Geometry check sheet. Reference: the model listing, model coordinates, mm. A direction names the side the tool comes from. Coordinates: 2 decimals unless noted, no trailing zeros. Order: outer loops, then holes, each group sorted by start corner. A loop starts at its lowest first (then second) coordinate and runs counter-clockwise, first axis right, second up. Notation, with made-up numbers: (77, 18) -> (118, 18) arc R16 cw to (118, 41) -> close; hole circle Ø8 at (-26, -24.75). An arc over 180 degrees is marked (long way). Answer as CSV lines item,"result". Start each with the question number.
from build123d import *

# Parameters (mm, degrees)
CROQUIS1_R                   = 3
SALIENTE_EXTRUIR1_DEPTH      = 5
SALIENTE_EXTRUIR2_DEPTH      = 16
SALIENTE_EXTRUIR3_DEPTH      = 3
SALIENTE_EXTRUIR3_DEPTH_BACK = 3
SALIENTE_EXTRUIR4_DEPTH      = 3
SALIENTE_EXTRUIR4_DEPTH_BACK = 3
REDONDEO1_R                  = 3


with BuildPart() as part:
    # Croquis1 → Saliente-Extruir1 (new body)
    with BuildSketch(Plane.XY):
        with BuildLine():
            Line((-8, 0), (-8, 45))
            Line((-8, 45), (8, 45))
            Line((8, 45), (8, 0))
            ThreePointArc((8, 0), (0, -8), (-8, 0))
        make_face()
        Circle(CROQUIS1_R, mode=Mode.SUBTRACT)
    extrude(amount=SALIENTE_EXTRUIR1_DEPTH)

    # Croquis2 → Saliente-Extruir2 (add)
    with BuildSketch(Plane.ZY.offset(8)):
        Polygon((5, 45), (95.630778704, 2.738173826), (94.098689817, -0.547401393), (5, 41), align=None)
    extrude(amount=-SALIENTE_EXTRUIR2_DEPTH)

    # Croquis3 → Saliente-Extruir3 (add, two sides)
    with BuildSketch(Plane(origin=(0, 0, 0), x_dir=(0, 0, -1), z_dir=(1, 0, 0))) as saliente_extruir3_sk:
        Polygon((-5, 11), (-50.315389352, 19.869086913), (-39.541185822, 24.893180529), (-5, 18.132810961), align=None)
    extrude(amount=SALIENTE_EXTRUIR3_DEPTH)
    extrude(saliente_extruir3_sk.sketch, amount=-SALIENTE_EXTRUIR3_DEPTH_BACK)

    # Croquis4 → Saliente-Extruir4 (add, two sides)
    with BuildSketch(Plane(origin=(0, 0, 0), x_dir=(0, 0, -1), z_dir=(1, 0, 0))) as saliente_extruir4_sk:
        Polygon((-95.630778704, 2.738173826), (-100.702197845, 13.61386727), (-78.044503169, 24.179323814), (-72.973084028, 13.303630369), align=None)
        with BuildLine():
            Line((-79.225631642, 13.698153291), (-91.91394066, 7.781497627))
            ThreePointArc((-91.91394066, 7.781497627), (-95.900718807, 9.232566203), (-94.449650231, 13.219344349))
            Line((-94.449650231, 13.219344349), (-81.761341212, 19.136000013))
            ThreePointArc((-81.761341212, 19.136000013), (-77.774563066, 17.684931437), (-79.225631642, 13.698153291))
        make_face(mode=Mode.SUBTRACT)
    extrude(amount=SALIENTE_EXTRUIR4_DEPTH)
    extrude(saliente_extruir4_sk.sketch, amount=-SALIENTE_EXTRUIR4_DEPTH_BACK)

    # Redondeo1
    redondeo1_edges = [part.edges().sort_by_distance(p)[0] for p in [
        (0, 13.61386727, 100.702197845),
        (0, 24.179323814, 78.044503169),
        (0, 45, 0),
    ]]
    fillet(redondeo1_edges, radius=REDONDEO1_R)


solid = part.part
Q1. Sectioned sample at D-D, the plane x = -5. Record the cut outline in (y, z) (3 decimals).
Q2. Sectioned sample at A-A, the plane x = 0. Record the cut outline in (y, z).
Q3. Access from +Z, -Z, +X, -X, +Y, -Y to the whole of each face (thin tool, end or side, straight path). Record for faces 1 (the cylindrical face through (-3, 0, 2)), 2 (the flat face through (0.04, 10.78, 85.48)), 3 (the flat face through (0.042, 15.372, 27.34)).
Q4. Sectioned sample at B-B, the plane z = 8. Record the cut outline in (x, y).
Q5. Thickness scan on L1, parallel to Y at x = 0, z = 3.25; L2, parallel to Y at x = 0, z = 2; L3, parallel to Z at x = -4, y = 17.5. Record the ranges inside material, lowest first.
Q6. Release check for a two-part mould opening along Y. For faces 4 (the flat face through (-3.668, 19.935, 50.173)), 5 (the flat face through (3, 18, 27)), 6 (the cylindrical face through (0.11, 44.1, 0.86)) record: released by +Y, released by -Y, zero draft, split by the parting line, or undercut.
Q7. Go/stop test with flat-tipped pins: pin 1 Ø3.5 at (x, y) = (0, 0) entering from -Z; pin 2 Ø5 at (y, z) = (9, 12.5) entering from -X; pin 3 Ø15.5 at (y, z) = (14.5, 37.5) entering from -X; pin 4 Ø1 at (x, z) = (4.5, 59.5) entering from +Y. Record where each tip stops, or that it passes through.
Q8. Sectioned sample at C-C, the plane y = 37.5. Record the cut outline in (x, z), then the cut area to 3 significant figures.
Geometry results:
1,outline,"(-6.245, 0) -> (42, 0) arc R3 ccw to (45, 3) -> (45, 5) -> (2.738, 95.631) -> (-0.547, 94.099) -> (41, 5) -> (-6.245, 5) -> close"
2,outline,"(-8, 0) -> (-3, 0) -> (-3, 5) -> (-8, 5) -> close; (-0.55, 94.1) -> (19.87, 50.32) -> (11, 5) -> (3, 5) -> (3, 0) -> (42, 0) arc R3 ccw to (45, 3) -> (45, 5) -> (13.3, 72.97) -> (21.46, 76.78) arc R3 ccw to (22.91, 80.76) -> (14.88, 97.98) arc R3 ccw to (10.89, 99.43) -> close; hole (7.78, 91.91) -> (13.7, 79.23) arc R3 ccw to (19.14, 81.76) -> (13.22, 94.45) arc R3 ccw to start; hole (18.13, 5) -> (41, 5) -> (24.89, 39.54) -> close"
3,face 1,"-Z"
3,face 2,"+X, -X"
3,face 3,"+X, -X, -Y"
4,outline,"(-8, 39.6) -> (8, 39.6) -> (8, 43.6) -> (-8, 43.6) -> close; (-3, 11.59) -> (3, 11.59) -> (3, 18.72) -> (-3, 18.72) -> close"
5,L1,"y = -8 to -3, 3 to 45"
5,L2,"y = -8 to -3, 3 to 44.83"
5,L3,"z = 0 to 5, 55.4 to 63.97"
6,face 4,"undercut"
6,face 5,"zero draft"
6,face 6,"released by +Y"
7,pin 1,"stops at z = 89.17"
7,pin 2,"passes through"
7,pin 3,"stops at x = -3"
7,pin 4,"stops at y = 19.82"
8,outline,"(-8, 0) -> (8, 0) -> (8, 5) -> (-8, 5) -> close; (-8, 12.51) -> (8, 12.51) -> (8, 21.08) -> (-8, 21.08) -> close"
8,area,"217 mm^2"
